Design review of the part built by this model. Coordinates are the model's own, in mm. Face numbers are marked on the shaded views. Give positions to 0.01 mm unless a question says otherwise; leave off trailing zeros. Loops run counter-clockwise (first coordinate to the right, second up) from the corner with the lowest first, then second, coordinate; pieces in that order, holes last. Notation, with made-up numbers: (0, 78) - (6, 78) arc R14 cw to (6, 101) - close; hole circle Ø9 at (72.5, -13.75). An arc over 180 degrees is marked (long way). Write each question's results on one line, items separated by ' | '.
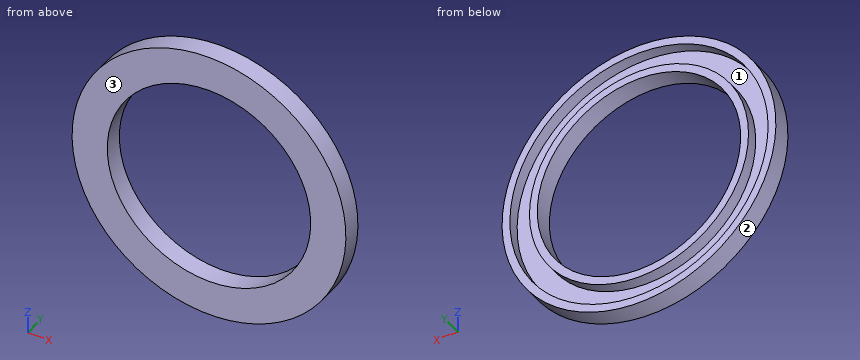
```python
from build123d import *

# Parameters (mm, degrees)
SKETCH_1_R          = 17.5
EXTRUDE_1_DEPTH     = 2.5
SKETCH_2_R          = 13
CUT_EXTRUDE_1_DEPTH = 2.5
SKETCH_3_R          = 16.5
SKETCH_3_R_2        = 14
CUT_EXTRUDE_2_DEPTH = 1.5


with BuildPart() as part:
    # 草图1 → 凸台-拉伸1 (new body)
    with BuildSketch(Plane(origin=(0, 0, 0), x_dir=(1, 0, 0), z_dir=(0, 1, 0))):
        with Locations(Location((0, 0, 0), (0, 0, 270))):
            Circle(SKETCH_1_R)
    extrude(amount=EXTRUDE_1_DEPTH)

    # 草图2 → 切除-拉伸1 (cut)
    with BuildSketch(Plane(origin=(0, 2.5, 0), x_dir=(1, 0, 0), z_dir=(0, 1, 0))):
        with Locations(Location((0, 0, 0), (0, 0, 270))):
            Circle(SKETCH_2_R)
    extrude(amount=-CUT_EXTRUDE_1_DEPTH, mode=Mode.SUBTRACT)

    # 草图3 → 切除-拉伸2 (cut)
    with BuildSketch(Plane(origin=(0, 2.5, 0), x_dir=(1, 0, 0), z_dir=(0, 1, 0))):
        with Locations(Location((0, 0, 0), (0, 0, 270))):
            Circle(SKETCH_3_R)
        with Locations(Location((0, 0, 0), (0, 0, 270))):
            Circle(SKETCH_3_R_2, mode=Mode.SUBTRACT)
    extrude(amount=-CUT_EXTRUDE_2_DEPTH, mode=Mode.SUBTRACT)


solid = part.part
```
Item 1: Clearance check with a flat-ended pin moving along its axis: P1, Ø1, axis at y = 2, z = 4, coming from the -X side. State where the tip first meets the part, or that it passes through.
Output values:
P1: stops at x = -17.15
Item 2: We need section A-A on x = 0. Give the boundary of the cut face in (y, z).
Output values:
outline: (0, -17.5) - (2.5, -17.5) - (2.5, -16.5) - (1, -16.5) - (1, -14) - (2.5, -14) - (2.5, -13) - (0, -13) - close; (0, 13) - (2.5, 13) - (2.5, 14) - (1, 14) - (1, 16.5) - (2.5, 16.5) - (2.5, 17.5) - (0, 17.5) - close
Item 3: We need section D-D on x = 14.5. Give the boundary of the cut face in (y, z), then the cut area to 3 significant figures.
Output values:
outline: (0, -9.8) - (2.5, -9.8) - (2.5, -7.87) - (1, -7.87) - (1, 7.87) - (2.5, 7.87) - (2.5, 9.8) - (0, 9.8) - close | area: 25.4 mm²
Item 4: Wall thickness on probe 1 along X at (y, z) = (1.85, 0); probe 2 along Z at (x, y) = (7, 2.35); probe 3 along Z at (x, y) = (1.5, 2.3): over which ranges is each line inside the solid? List them lowest first.
Output values:
probe 1: x = -17.5 to -16.5, -14 to -13, 13 to 14, 16.5 to 17.5 | probe 2: z = -16.04 to -14.94, -12.12 to -10.95, 10.95 to 12.12, 14.94 to 16.04 | probe 3: z = -17.44 to -16.43, -13.92 to -12.91, 12.91 to 13.92, 16.43 to 17.44
Item 5: Draft analysis for pull direction X (two halves, no side actions). For the marked faces 1, 2 and 3, state which applies: +X half, -X half, draft (parallel to the pull), parting line (faces both ways), or undercut.
Output values:
face 1: undercut | face 2: parting line | face 3: draft
Item 6: We need section B-B on z = 0. Give the boundary of the cut face in (x, y).
Output values:
outline: (-17.5, 0) - (-13, 0) - (-13, 2.5) - (-14, 2.5) - (-14, 1) - (-16.5, 1) - (-16.5, 2.5) - (-17.5, 2.5) - close; (13, 0) - (17.5, 0) - (17.5, 2.5) - (16.5, 2.5) - (16.5, 1) - (14, 1) - (14, 2.5) - (13, 2.5) - close
Item 7: We need section C-C on y = 1.4. Give the boundary of the cut face in (x, z), then the cut area to 3 significant figures.
Output values:
outline: circle Ø35 at (0, 0); circle Ø28 at (0, 0); hole circle Ø33 at (0, 0); hole circle Ø26 at (0, 0) | area: 192 mm²
